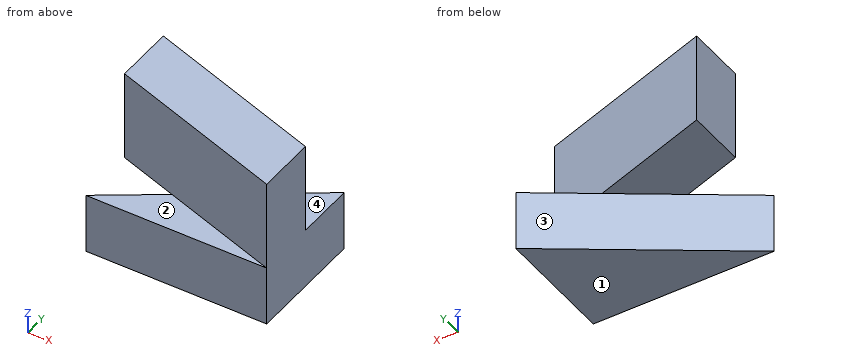
from build123d import *

# Parameters (mm, degrees)
BOSS_EXTRUDE1_DEPTH = 10
BOSS_EXTRUDE2_DEPTH = 15


with BuildPart() as part:
    # Sketch1 → Boss-Extrude1 (new body)
    with BuildSketch(Plane.XY):
        Polygon((-30, 0), (0, 0), (0, 20), align=None)
    extrude(amount=BOSS_EXTRUDE1_DEPTH)

    # Sketch2 → Boss-Extrude2 (add)
    with BuildSketch(Plane.XY.offset(10)):
        Polygon((0, 10), (0, 0), (-30, 10), (-30, 20), align=None)
    extrude(amount=BOSS_EXTRUDE2_DEPTH)


solid = part.part
Geometry: final body of the model. Coordinates: model frame, mm. Face numbers are marked on the shaded views. A direction names the side the tool comes from. Give positions to 0.01 mm unless a question says otherwise; leave off trailing zeros. Loops run counter-clockwise (first coordinate to the right, second up) from the corner with the lowest first, then second, coordinate; pieces in that order, holes last. Notation, with made-up numbers: M 80.25,-4 L 101.25,-4 A12 cw 101.25,9 Z; hole C 78,-3 d8. An arc over 180 degrees is marked long. Put each result on its own line as item: value.
1) Cut plane D-D, the plane x = -13.5. Return the cut outline in (y, z).
Computed values:
outline: M 0,0 L 11,0 L 11,10 L 14.5,10 L 14.5,25 L 4.5,25 L 4.5,10 L 0,10 Z
2) Cut plane C-C, the plane y = 10.5. Return the cut outline in (x, z), plus the area to 3 significant figures.
Computed values:
outline: M -30,10 L -14.25,10 L -14.25,0 L 0,0 L 0,10 L -1.5,10 L -1.5,25 L -30,25 Z
area: 570 mm^2
3) Material intervals for L1, parallel to Z at x = -24, y = 9.75; L2, parallel to Y at x = -13, z = 8; L3, parallel to X at y = 2, z = 1.75, sorted ascending. Write a range as from..to.
Computed values:
L1: z = 10..25
L2: y = 0..11.33
L3: x = -27..0
4) Reachability of the marked faces 1, 2, 3 and 4 from +Z, -Z, +X, -X, +Y, -Y: full face, straight path, thin tool, end or side. Return the list, or none.
Computed values:
face 1: -Z, +X, -X, +Y, -Y
face 2: +Z, -X, -Y
face 3: -Z, -X, +Y
face 4: +Z, +X, +Y
5) Cut plane B-B, the plane x = -25. Return the cut outline in (y, z), plus the area to 3 significant figures.
Computed values:
outline: M 0,0 L 3.33,0 L 3.33,10 L 0,10 Z; M 8.33,10 L 18.33,10 L 18.33,25 L 8.33,25 Z
area: 183 mm^2
6) Cut plane A-A, the plane y = 14.5. Return the cut outline in (x, z), plus the area to 3 significant figures.
Computed values:
outline: M -30,10 L -13.5,10 L -13.5,25 L -30,25 Z; M -8.25,0 L 0,0 L 0,10 L -8.25,10 Z
area: 330 mm^2
7) First-contact query: P1, Ø4, axis at y = 10, z = 7, coming from the -X side; P2, Ø8, axis at x = -23.5, z = 5, coming from the +Y side; P3, Ø8, axis at x = -16.5, z = 18.5, coming from the +Y side. Flat tips, straight axial feed; report the tip coordinate or a pass-through.
Computed values:
P1: stops at x = -18
P2: stops at y = 7
P3: stops at y = 16.83
